Verification items for the finished model (mm, model axes). Face numbers are marked on the shaded views. Coordinates: 2 decimals unless noted, no trailing zeros. Order: outer loops, then holes, each group sorted by start corner. A loop starts at its lowest first (then second) coordinate and runs counter-clockwise, first axis right, second up. Notation, with made-up numbers: M 67,15.25 L 118,15.25 A24 ccw 118,39.25 Z; hole C 76.25,74 d11. An arc over 180 degrees is marked long. Return JSON: item names as keys, results as strings. Group by question number.
1. Section check A-A, the plane y = -26.5. Record the cut outline in (x, z).
2. Section check C-C, the plane x = 141.5. Record the cut outline in (y, z), plus the area to 3 significant figures.
3. Gauge pin test, flat ends, axial feed: pin 1 (0.7 mm diameter, centred on x = 472.5, y = -21, fed in from +Z); pin 2 (2 mm diameter, centred on x = -93.5, z = -201, fed in from -Y). Record the tip position at first contact, or that the pin passes through.
4. Material ranges on line 1 along X through (y, z) = (-9.5, -13); line 2 along Y through (x, z) = (191.5, -533), recorded low to high.
5. Mould release check, pull along X, two halves, no side actions. Record for the marked faces 1 and 2: +X half, -X half, draft (parallel to the pull), parting line (faces both ways), or undercut.
6. Section check B-B, the plane z = -48. Record the cut outline in (x, y).
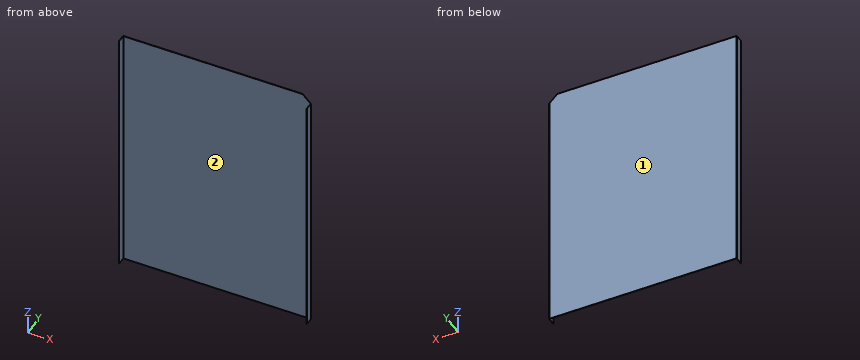
```python
from build123d import *

# Parameters (mm, degrees)
SKETCH1_W                      = 947.4
SKETCH1_H                      = 1277.4
BASE_FLANGE1_DEPTH             = 1.2
CUT_EXTRUDE1_DEPTH             = 10
EDGE_FLANGE1_STRIP_W           = 7.2
EDGE_FLANGE1_STRIP_H           = 1.2
EDGE_FLANGE1_STRIP_CUT_DEPTH   = 1236.2
EDGE_FLANGE1_STRIP_2_W         = 7.2
EDGE_FLANGE1_STRIP_2_H         = 1.2
EDGE_FLANGE1_STRIP_CUT_2_DEPTH = 1277.4
EDGE_FLANGE1_DEPTH             = 1236.2
EDGE_FLANGE1_BEND_DEPTH        = 1277.4


# Sheet-metal steps are written as plain solids
with BuildPart() as part:
    # Sketch1 → Base-Flange1 (new body)
    with BuildSketch(Plane(origin=(0, 0, 0), x_dir=(1, 0, 0), z_dir=(0, 1, 0))):
        Rectangle(SKETCH1_W, SKETCH1_H)
    extrude(amount=-BASE_FLANGE1_DEPTH)

    # Sketch3 → Cut-Extrude1 (cut)
    with BuildSketch(Plane.XZ.offset(1.2)):
        Polygon((431.3, 638.7), (512.405547978, 658.605547978), (473.7, 597.5), align=None)
    extrude(amount=-CUT_EXTRUDE1_DEPTH, mode=Mode.SUBTRACT)

    # Edge-Flange1 strip (across the edge) → Edge-Flange1 strip cut (cut)
    with BuildSketch(Plane(origin=(473.7, -1.2, -638.7), x_dir=(-1, 0, 0), z_dir=(0, 0, 1))):
        with Locations((-1.2, -0.6)):
            Rectangle(EDGE_FLANGE1_STRIP_W, EDGE_FLANGE1_STRIP_H)
    extrude(amount=EDGE_FLANGE1_STRIP_CUT_DEPTH, mode=Mode.SUBTRACT)

    # Edge-Flange1 strip 2 (across the edge) → Edge-Flange1 strip cut 2 (cut)
    with BuildSketch(Plane(origin=(-473.7, -1.2, 638.7), x_dir=(1, 0, 0), z_dir=(0, 0, -1))):
        with Locations((-1.2, -0.6)):
            Rectangle(EDGE_FLANGE1_STRIP_2_W, EDGE_FLANGE1_STRIP_2_H)
    extrude(amount=EDGE_FLANGE1_STRIP_CUT_2_DEPTH, mode=Mode.SUBTRACT)

    # Edge-Flange1 section (across the edge) → Edge-Flange1 (add)
    with BuildSketch(Plane(origin=(473.7, -1.2, -638.7), x_dir=(-1, 0, 0), z_dir=(0, 0, 1))):
        with BuildLine():
            Line((0, 1.2), (0, 40))
            Line((0, 40), (1.2, 40))
            Line((1.2, 40), (1.2, 1.2))
            ThreePointArc((1.2, 1.2), (1.551471863, 0.351471863), (2.4, 0))
            Line((2.4, 0), (2.4, -1.2))
            ThreePointArc((2.4, -1.2), (0.702943725, -0.497056275), (0, 1.2))
        make_face()
    extrude(amount=EDGE_FLANGE1_DEPTH)

    # Edge-Flange1 section 2 (across the edge) → Edge-Flange1 bend (add)
    with BuildSketch(Plane(origin=(-473.7, -1.2, 638.7), x_dir=(1, 0, 0), z_dir=(0, 0, -1))):
        with BuildLine():
            Line((0, 1.2), (0, 40))
            Line((0, 40), (1.2, 40))
            Line((1.2, 40), (1.2, 1.2))
            ThreePointArc((1.2, 1.2), (1.551471863, 0.351471863), (2.4, 0))
            Line((2.4, 0), (2.4, -1.2))
            ThreePointArc((2.4, -1.2), (0.702943725, -0.497056275), (0, 1.2))
        make_face()
    extrude(amount=EDGE_FLANGE1_BEND_DEPTH)


solid = part.part
```
Answers follow:
{
 "1": {"outline": "M -473.7,-638.7 L -472.5,-638.7 L -472.5,638.7 L -473.7,638.7 Z; M 472.5,-638.7 L 473.7,-638.7 L 473.7,597.5 L 472.5,597.5 Z"},
 "2": {"outline": "M -1.2,-638.7 L 0,-638.7 L 0,638.7 L -1.2,638.7 Z", "area": "1,530 mm^2"},
 "3": {"pin 1": "z = 597.5", "pin 2": "y = -1.2"},
 "4": {"line 1": "-473.7 to -472.5, 472.5 to 473.7", "line 2": "-1.2 to 0"},
 "5": {"face 1": "draft", "face 2": "undercut"},
 "6": {"outline": "M -473.7,-41.2 L -472.5,-41.2 L -472.5,-2.4 A1.2 cw -471.3,-1.2 L 471.3,-1.2 A1.2 cw 472.5,-2.4 L 472.5,-41.2 L 473.7,-41.2 L 473.7,-2.4 A2.4 ccw 471.3,0 L -471.3,0 A2.4 ccw -473.7,-2.4 Z"}
}
